Build history of the part. All positions in model axes, mm. A direction names the side the tool comes from. Coordinates: 2 decimals unless noted, no trailing zeros. Loops run counter-clockwise (first coordinate to the right, second up) from the corner with the lowest first, then second, coordinate; pieces in that order, holes last.
Item 1: 3-axis set-ups, long thin cutter, end or side, ignore diameter. For faces 5 (the face through (4.507, 66.683, 0.26)), 6 (the face through (0, 39, -4)): which of +Z, -Z, +X, -X, +Y, -Y reach the whole face in a straight line?
Item 2: Cut at B-B (y = 35.5). List the corners of the cut face in (x, z).
Item 3: Cut at A-A (x = 2.5). List the corners of the cut face in (y, z), and give its area (3 significant figures).
Item 4: Cut at D-D (y = 76.2). List the corners of the cut face in (x, z), and give its area (3 significant figures).
Item 5: Cut at C-C (z = 0). Count the separate pieces of the cut face and the enclosed holes in it, and give its area (3 significant figures).
Item 6: Mould opens along Z. For faces 1 (the face through (0, 39, 5)), 2 (the face through (-4.5, 0, -0.1)), 3 (the face through (4.51, 5.07, 1.5)), 4 (the face through (0, 39, -5)) say: released by +Z, released by -Z, zero draft, split by the parting line, or undercut.
Item 7: Flat gauge pin, fed straight in: pin 1 (1.8 mm diameter, centred on x = 0, y = 66.7, fed in from -Z). Where does the tip first touch, or does it go through?
Item 8: Drill centre lines: line 1 along Y through (x, z) = (0, 4.3); line 2 along X through (y, z) = (63, 3.5). Where is each one in solid material? Low to high.
from build123d import *

# Parameters (mm, degrees)
SKETCH_1_W          = 10
SKETCH_1_H          = 10
SKETCH_1_W_2        = 8
SKETCH_1_H_2        = 8
EXTRUDE_1_DEPTH     = 104.9
SKETCH_2_R          = 1.6
SKETCH_2_R_2        = 1.5
CUT_EXTRUDE_1_DEPTH = 106.494123059
SKETCH_3_R          = 1.5
SKETCH_3_R_2        = 2
CUT_EXTRUDE_2_DEPTH = 106.494123059
SKETCH_4_W          = 10
SKETCH_4_H          = 10
CUT_EXTRUDE_3_DEPTH = 25


with BuildPart() as part:
    # ｽｹｯﾁ1 → 押し出し-薄板1 (new body)
    with BuildSketch(Plane(origin=(0, 0, 0), x_dir=(1, 0, 0), z_dir=(0, 1, 0))):
        Rectangle(SKETCH_1_W, SKETCH_1_H)
        Rectangle(SKETCH_1_W_2, SKETCH_1_H_2, mode=Mode.SUBTRACT)
    extrude(amount=EXTRUDE_1_DEPTH)

    # ｽｹｯﾁ2 → ｶｯﾄ - 押し出し1 (cut, through all)
    with BuildSketch(Plane.XY.offset(5)):
        with Locations((0, 5)):
            Circle(SKETCH_2_R)
        with Locations((0, 15)):
            Circle(SKETCH_2_R)
        with Locations((0, 92.95)):
            Circle(SKETCH_2_R_2)
        with Locations((0, 66.7)):
            Circle(SKETCH_2_R_2)
        with Locations((0, 99.9)):
            Circle(SKETCH_2_R_2)
    extrude(amount=-CUT_EXTRUDE_1_DEPTH, mode=Mode.SUBTRACT)

    # ｽｹｯﾁ3 → ｶｯﾄ - 押し出し2 (cut, through all)
    with BuildSketch(Plane(origin=(5, 0, 0), x_dir=(0, 0, -1), z_dir=(1, 0, 0))):
        with Locations((0, 76.2)):
            Circle(SKETCH_3_R)
        with Locations((0, 5)):
            Circle(SKETCH_3_R)
        with Locations((0, 64.7)):
            Circle(SKETCH_3_R_2)
        with Locations((0, 29.7)):
            Circle(SKETCH_3_R_2)
        with Locations((0, 48.2)):
            Circle(SKETCH_3_R)
        with Locations((0, 56.2)):
            Circle(SKETCH_3_R)
    extrude(amount=-CUT_EXTRUDE_2_DEPTH, mode=Mode.SUBTRACT)

    # ｽｹｯﾁ4 → ｶｯﾄ - 押し出し3 (cut)
    with BuildSketch(Plane(origin=(0, 104.9, 0), x_dir=(1, 0, 0), z_dir=(0, 1, 0))):
        Rectangle(SKETCH_4_W, SKETCH_4_H)
    extrude(amount=-CUT_EXTRUDE_3_DEPTH, mode=Mode.SUBTRACT)


solid = part.part
Filled sheet:
1. face 5: +X, -X
1. face 6: +Y, -Y
2. outline: (-5, -5) - (5, -5) - (5, 5) - (-5, 5) - close; hole (-4, -4) - (4, -4) - (4, 4) - (-4, 4) - close
3. outline: (0, -5) - (79.9, -5) - (79.9, -4) - (0, -4) - close; (0, 4) - (79.9, 4) - (79.9, 5) - (0, 5) - close
3. area: 160 mm2
4. outline: (-5, -5) - (5, -5) - (5, -1.5) - (4, -1.5) - (4, -4) - (-4, -4) - (-4, -1.5) - (-5, -1.5) - close; (-5, 1.5) - (-4, 1.5) - (-4, 4) - (4, 4) - (4, 1.5) - (5, 1.5) - (5, 5) - (-5, 5) - close
4. area: 30.0 mm2
5. separate pieces: 14
5. enclosed holes: 0
5. area: 120 mm2
6. face 1: released by +Z
6. face 2: zero draft
6. face 3: undercut
6. face 4: released by -Z
7. pin 1: passes through
8. line 1: y = 0 to 3.4, 6.6 to 13.4, 16.6 to 65.2, 68.2 to 79.9
8. line 2: x = -5 to -4, 4 to 5
